Autodesk Inventor part; units mm, degrees
ref_plane "YZ Plane" through (0, 0, 0) normal (1, 0, 0) x (0, 1, 0)
ref_plane "XZ Plane" through (0, 0, 0) normal (0, 1, 0) x (-1, 0, 0)
ref_plane "XY Plane" through (0, 0, 0) normal (0, 0, 1) x (1, 0, 0)
sketch "Sketch1" plane through (0, 0, 0) normal (0, 0, 1) x (1, 0, 0)
  line L0 (0, 0) -> (495.3, 0)
  line L1 (495.3, 0) -> (495.3, 158.75)
  line L2 (495.3, 190.5) -> (457.2, 190.5) construction
  line L3 (0, 190.5) -> (0, 158.75) construction
  arc A0 (25.4, 158.75) -> (38.1, 171.45) centre (25.4, 171.45) ccw
  arc A1 (457.2, 171.45) -> (469.9, 158.75) centre (469.9, 171.45) ccw
  line L4 (25.4, 158.75) -> (0, 158.75)
  line L5 (38.1, 171.45) -> (38.1, 190.5)
  line L6 (469.9, 158.75) -> (495.3, 158.75)
  line L7 (457.2, 171.45) -> (457.2, 190.5)
  line L8 (38.1, 190.5) -> (0, 190.5) construction
  line L9 (0, 158.75) -> (0, 0)
  line L10 (457.2, 190.5) -> (38.1, 190.5)
  line L11 (495.3, 158.75) -> (495.3, 190.5) construction
  dimension "d0" = 190.5
  dimension "d1" = 495.3
  dimension "d4" = 25.4
  dimension "d5" = 25.4
  dimension "d6" = 25.4
  dimension "d7" = 19.05
  dimension "d8" = 25.4
  dimension "d9" = 19.05
extrude "Extrusion1" add sketch "Sketch1" against normal blind 6.35
equation "\"d5\" = d4"
equation "\"d8\" = d6"
equation "\"d9\" = d7"
properties part number "manipulator side pannel"
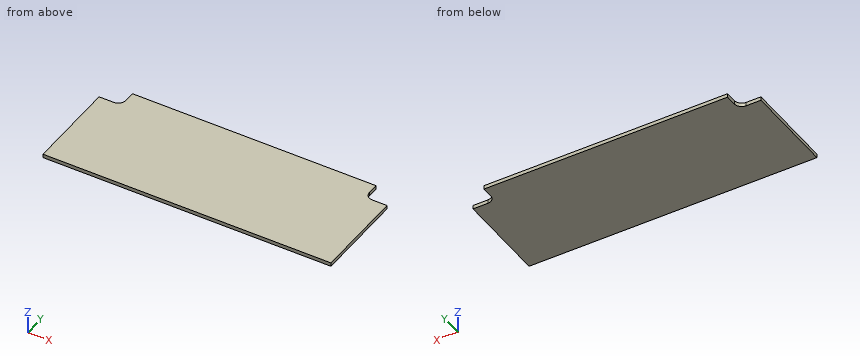
Build history of the part. All positions in model axes, mm. Give positions to 0.01 mm unless a question says otherwise; leave off trailing zeros. Order: outer loops, then holes, each group sorted by start corner. A loop starts at its lowest first (then second) coordinate and runs counter-clockwise, first axis right, second up. Notation, with made-up numbers: M 89,-16.75 L 93,-16.75 A18 cw 93,7.25 Z; hole C 76,-30.5 d1. An arc over 180 degrees is marked long. Return JSON: item names as keys, results as strings.
Q1. Wall check: probe 1 along X at (y, z) = (176.5, -5.75); probe 2 along X at (y, z) = (166, -4.25). Give the ranges that are in metal, low to high. Write a range as from..to.
Answer list:
{"probe 1": "x = 38.1..457.2", "probe 2": "x = 36.87..458.43"}
Q2. Band-saw the part on A-A (z = -2). Give the cut face in (x, y), then the cut area to 3 significant figures.
Answer list:
{"outline": "M 0,0 L 495.3,0 L 495.3,158.75 L 469.9,158.75 A12.7 cw 457.2,171.45 L 457.2,190.5 L 38.1,190.5 L 38.1,171.45 A12.7 cw 25.4,158.75 L 0,158.75 Z", "area": "92,000 mm^2"}
Q3. Flat gauge pins, fed straight in: pin 1 (1.9 mm diameter, centred on y = 178.5, z = -2.5, fed in from +X); pin 2 (3 mm diameter, centred on x = 488, z = -3.5, fed in from +Y). Where does each tip first touch, or does it go through?
Answer list:
{"pin 1": "stops at x = 457.2", "pin 2": "stops at y = 158.75"}
